The listing builds one solid part. Answer for the finished solid, in the listing's coordinates (mm). Face numbers are marked on the shaded views. Coordinates: 2 decimals unless noted, no trailing zeros. Loops run counter-clockwise (first coordinate to the right, second up) from the corner with the lowest first, then second, coordinate; pieces in that order, holes last. Notation, with made-up numbers: M 60,45.25 L 111,45.25 A32 cw 111,75.25 Z; hole C -32,-34 d5. An arc over 180 degrees is marked long. Answer as a JSON object with one key per item and string values. Group by question number.
1. Given pin 1 (1 mm diameter, centred on x = -1, z = -8.5, fed in from -Y); pin 2 (0.5 mm diameter, centred on y = -0.5, z = 13.5, fed in from +X); pin 3 (3 mm diameter, centred on x = 0, z = 8, fed in from +Y), each flat-ended and moving along its own axis, determine where each tip first touches the part or whether it passes through.
2. A cutting plane is placed at A-A on z = -3. Give the vertices of the cut face in (x, y).
3. Straight lines are drawn through the part: L1, parallel to Z at x = -1, y = 2; L2, parallel to Z at x = 0, y = -0.5; L3, parallel to Y at x = 1.5, z = 4. For each, find the intervals that lie inside material, in ascending order.
4. Determine the mould class of the marked faces 1, 2 and 3 for opening direction X: released by +X, released by -X, zero draft, split by the parting line, or undercut.
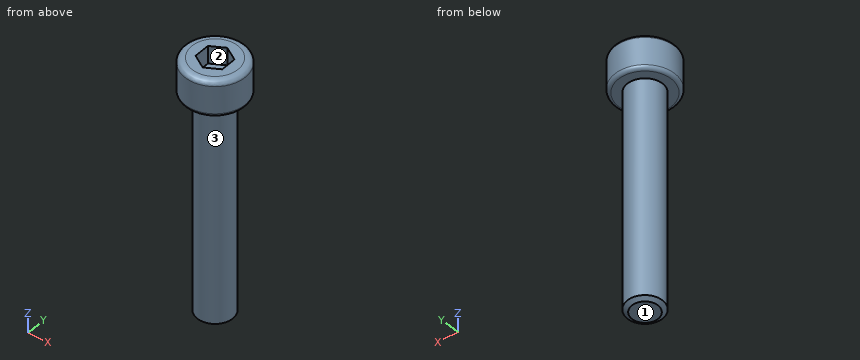
from build123d import *

# Parameters (mm, degrees)
CHAMFER_1_SIZE      = 0.3
CHAMFER_1_SIZE2     = 0.519615242
FILLET_1_R          = 0.4
FILLET_2_SIZE       = 0.5
FILLET_2_SIZE_2     = 0.8
CUT_EXTRUDE_1_DEPTH = 2


with BuildPart() as part:
    # 草图2 → 旋转1 (revolve)
    with BuildSketch(Plane(origin=(0, 0, 0), x_dir=(0, 0, -1), z_dir=(1, 0, 0)), mode=Mode.PRIVATE) as revolve_1_sk:
        Polygon((-14.5, 0), (-14.5, 3.4), (-10.5, 3.4), (-10.5, 2), (14.5, 2), (14.5, 0), align=None)
    revolve(revolve_1_sk.sketch.rotate(Axis((0, 0, -14.5), (0, 0, 1)), 90), axis=Axis((0, 0, -14.5), (0, 0, 1)))

    # 倒角1
    chamfer_1_edges = [part.edges().sort_by_distance(p)[0] for p in [
        (2, 0, -14.5),
    ]]
    chamfer_1_side = [part.faces().sort_by_distance(p)[0] for p in [
        (2, 0, -2),
    ]]
    chamfer(chamfer_1_edges, length=CHAMFER_1_SIZE, length2=CHAMFER_1_SIZE2, reference=chamfer_1_side[0])

    # 圆角1
    fillet_1_edges = [part.edges().sort_by_distance(p)[0] for p in [
        (3.4, 0, 10.5),
    ]]
    fillet(fillet_1_edges, radius=FILLET_1_R)

    # 圆角2
    # an asymmetric fillet: 0.8, 0.5 mm, written as the material it takes off along each edge
    with BuildSketch(Plane(origin=(0, 0, 14.5), x_dir=(-1, 0, 0), z_dir=(0, 1, 0))) as fillet_2_piece_1:
        with BuildLine():
            Bezier((3.4, -FILLET_2_SIZE), (3.4, 0), (3.4 - FILLET_2_SIZE_2, 0), weights=[1, 0.707106781, 1])
            Line((3.4 - FILLET_2_SIZE_2, 0), (3.4, 0))
            Line((3.4, 0), (3.4, -FILLET_2_SIZE))
        make_face()
    revolve(axis=Axis((0, 0, 14.5), (0, 0, 1)), mode=Mode.SUBTRACT)

    # 草图3 → 切除-拉伸1 (cut)
    with BuildSketch(Plane.XY.offset(14.5)):
        Polygon((0, 1.732050808), (-1.5, 0.866025404), (-1.5, -0.866025404), (0, -1.732050808), (1.5, -0.866025404), (1.5, 0.866025404), align=None)
    extrude(amount=-CUT_EXTRUDE_1_DEPTH, mode=Mode.SUBTRACT)


solid = part.part
From the geometry:
{
 "1": {"pin 1": "stops at y = -1.94", "pin 2": "stops at x = 3.39", "pin 3": "stops at y = 2"},
 "2": {"outline": "C 0,0 d4"},
 "3": {"L1": "z = 10.5 to 14.5", "L2": "z = -14.5 to 12.5", "L3": "y = -1.32 to 1.32"},
 "4": {"face 1": "zero draft", "face 2": "undercut", "face 3": "split by the parting line"}
}
